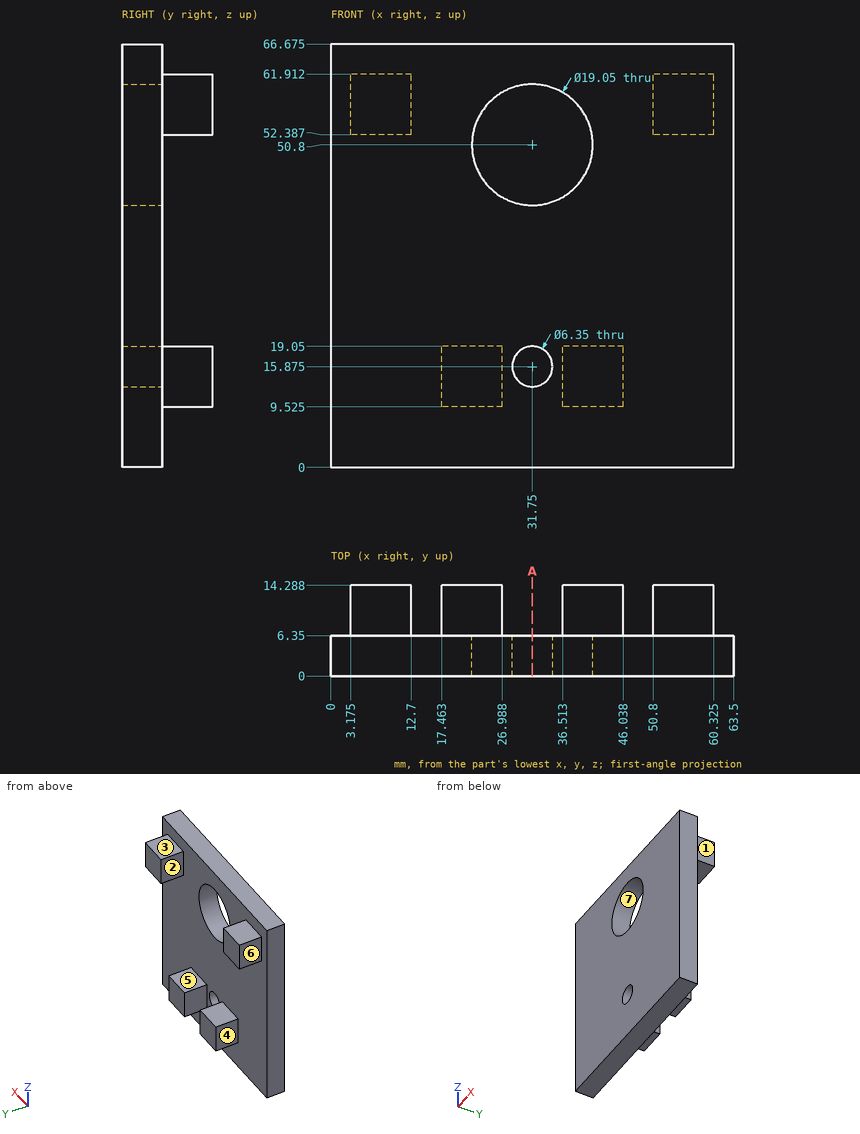
The drawing under review shows one solid part. Ordinate dimensions are in mm from its lowest x, y, z. A direction names the side the tool comes from. Give positions to 0.01 mm unless a question says otherwise; leave off trailing zeros. One line per item, written item: value. Start each with the question number.
Q1. Clearance check with flat-ended pins moving along their axes: pin 1 Ø4 at (x, y) = (16.5, 8.5) entering from +Z; pin 2 Ø1.5 at (y, z) = (9, 59.5) entering from -X (1 decimal); pin 3 Ø2.5 at (x, y) = (6, 10.5) entering from +Z. State where each tip first meets the part, or that it passes through.
Q2. For L1, parallel to Z at x = 31.5, y = 5.75 (1 decimal); L2, parallel to X at y = 11.75, z = 13.5; L3, parallel to Y at x = 9.5, z = 44, list the stretches that pass through material, from the lowest coordinate up.
Q3. Add section A-A (x = 31.75). Count the separate pieces of the cut face and the enclosed holes in it, and give its area (3 significant figures).
Q4. Draft analysis for pull direction Z (two halves, no side actions). For the marked faces 5, 6 and 7, state which applies: released by +Z, released by -Z, zero draft, split by the parting line, or undercut.
Q5. Machinability: for the marked faces 1, 2, 3 and 4, which of the approach directions +Z, -Z, +X, -X, +Y, -Y give a long, thin tool a straight path to every point of the face, cutting with its end or side? Answer none if there is none.
Reply:
1. pin 1: z = 19.05
1. pin 2: x = 3.2
1. pin 3: z = 61.91
2. L1: 0 to 12.7, 19 to 41.3, 60.3 to 66.7
2. L2: 17.46 to 26.99, 36.51 to 46.04
2. L3: 0 to 6.35
3. separate pieces: 3
3. enclosed holes: 0
3. area: 262 mm²
4. face 5: released by +Z
4. face 6: zero draft
4. face 7: undercut
5. face 1: +Z, -Z, +X, +Y
5. face 2: +Z, -Z, +Y
5. face 3: +Z, +X, -X, +Y
5. face 4: +Z, -Z, -X, +Y
